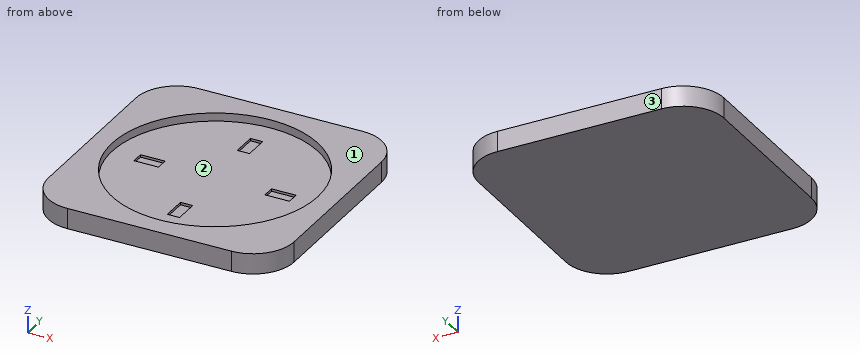
```python
from build123d import *

# Parameters (mm, degrees)
F0_W     = 60
F0_H     = 60
F1_DEPTH = 5
F2_R     = 25.12858
F3_DEPTH = 2
F4_R     = 10
F5_W     = 6
F5_H     = 3
F5_W_2   = 3
F5_H_2   = 6
F6_DEPTH = 0.6


with BuildPart() as f1:
    # F0 (on Top) → F1 (new body)
    with BuildSketch(Plane.XY):
        Rectangle(F0_W, F0_H)
    extrude(amount=F1_DEPTH)

    # F2 (on face) → F3 (cut)
    with BuildSketch(Plane.XY.offset(5)):
        Circle(F2_R)
    extrude(amount=-F3_DEPTH, mode=Mode.SUBTRACT)

    # F4
    f4_edges = [f1.edges().sort_by_distance(p)[0] for p in [
        (30, 30, 2.5),
        (30, -30, 2.5),
        (-30, -30, 2.5),
        (-30, 30, 2.5),
    ]]
    fillet(f4_edges, radius=F4_R)

    # F5 (on face) → F6 (cut)
    with BuildSketch(Plane.XY.offset(3)):
        with Locations((16, 0)):
            Rectangle(F5_W, F5_H)
        with Locations((0, 16)):
            Rectangle(F5_W_2, F5_H_2)
        with Locations((-16, 0)):
            Rectangle(F5_W, F5_H)
        with Locations((0, -16)):
            Rectangle(F5_W_2, F5_H_2)
    extrude(amount=-F6_DEPTH, mode=Mode.SUBTRACT)


solid = f1.part
```
The model under review builds one solid part; all positions refer to its coordinate system, in mm. Face numbers are marked on the shaded views. Give positions to 0.01 mm unless a question says otherwise; leave off trailing zeros. Write each loop counter-clockwise with the first axis right and the second up, starting at its lowest first coordinate (ties: lowest second). Pieces come first, ordered by that corner, then holes.
(1) To check wall thickness, follow L1, parallel to Y at x = 0, z = 3.85; L2, parallel to X at y = -17, z = 2.65; L3, parallel to Z at x = -10, y = -19. State the ranges of each line that lie inside material, in increasing order.
(2) Consider section D-D, the plane x = -17. Give the boundary of the cut face in (y, z).
(3) The part is to be moulded in two halves that separate along Y. For the marked faces 1, 2 and 3, say which applies: released by +Y, released by -Y, zero draft, split by the parting line, or undercut.
(4) Consider section B-B, the plane x = 0. Give the boundary of the cut face in (y, z).
(5) For P1, Ø1, axis at x = 3, y = -13, coming from the +Z side; P2, Ø0.9, axis at x = 0, y = 15, coming from the +Z side, all flat-tipped, find the tip position at first contact; note any pin that passes through.
(6) Consider section A-A, the plane z = 1.45. Give the boundary of the cut face in (x, y).
Returned:
1. L1: y = -30 to -25.13, 25.13 to 30
1. L2: x = -30 to -1.5, 1.5 to 30
1. L3: z = 0 to 3
2. outline: (-30, 0) - (30, 0) - (30, 5) - (18.51, 5) - (18.51, 3) - (1.5, 3) - (1.5, 2.4) - (-1.5, 2.4) - (-1.5, 3) - (-18.51, 3) - (-18.51, 5) - (-30, 5) - close
3. face 1: zero draft
3. face 2: undercut
3. face 3: released by +Y
4. outline: (-30, 0) - (30, 0) - (30, 5) - (25.13, 5) - (25.13, 3) - (19, 3) - (19, 2.4) - (13, 2.4) - (13, 3) - (-13, 3) - (-13, 2.4) - (-19, 2.4) - (-19, 3) - (-25.13, 3) - (-25.13, 5) - (-30, 5) - close
5. P1: stops at z = 3
5. P2: stops at z = 2.4
6. outline: (-30, -20) arc R10 ccw to (-20, -30) - (20, -30) arc R10 ccw to (30, -20) - (30, 20) arc R10 ccw to (20, 30) - (-20, 30) arc R10 ccw to (-30, 20) - close
